The listing builds one solid part. Answer for the finished solid, in the listing's coordinates (mm). Coordinates: 2 decimals unless noted, no trailing zeros. Order: outer loops, then holes, each group sorted by start corner. A loop starts at its lowest first (then second) coordinate and runs counter-clockwise, first axis right, second up.
from build123d import *

# Parameters (mm, degrees)
F0_W     = 133.35
F0_H     = 73.025
F1_DEPTH = 3.175
F2_R     = 3.175
F3_DEPTH = 3.176
F4_R     = 3.96875
F5_DEPTH = 3.176


with BuildPart() as f1:
    # F0 (on Top) → F1 (new body)
    with BuildSketch(Plane.XY):
        with Locations((66.675, 36.5125)):
            Rectangle(F0_W, F0_H)
    extrude(amount=-F1_DEPTH)

    # F2 (on face) → F3 (cut, through all)
    with BuildSketch(Plane(origin=(0, 0, -3.175), x_dir=(1, 0, 0), z_dir=(0, 0, -1))):
        with Locations((28.575, -36.5125)):
            Circle(F2_R)
        with Locations((53.975, -36.5125)):
            Circle(F2_R)
        with Locations((79.375, -36.5125)):
            Circle(F2_R)
        with Locations((104.775, -36.5125)):
            Circle(F2_R)
    extrude(amount=-F3_DEPTH, mode=Mode.SUBTRACT)

    # F4 (on face) → F5 (cut, through all)
    with BuildSketch(Plane(origin=(0, 0, -3.175), x_dir=(1, 0, 0), z_dir=(0, 0, -1))):
        with Locations((28.575, -54.79161)):
            Circle(F4_R)
        with Locations((53.975, -54.79161)):
            Circle(F4_R)
        with Locations((79.375, -54.79161)):
            Circle(F4_R)
        with Locations((104.775, -54.79161)):
            Circle(F4_R)
        with Locations((104.775, -18.27911)):
            Circle(F4_R)
        with Locations((79.375, -18.27911)):
            Circle(F4_R)
        with Locations((53.975, -18.27911)):
            Circle(F4_R)
        with Locations((28.575, -18.27911)):
            Circle(F4_R)
    extrude(amount=-F5_DEPTH, mode=Mode.SUBTRACT)


solid = f1.part
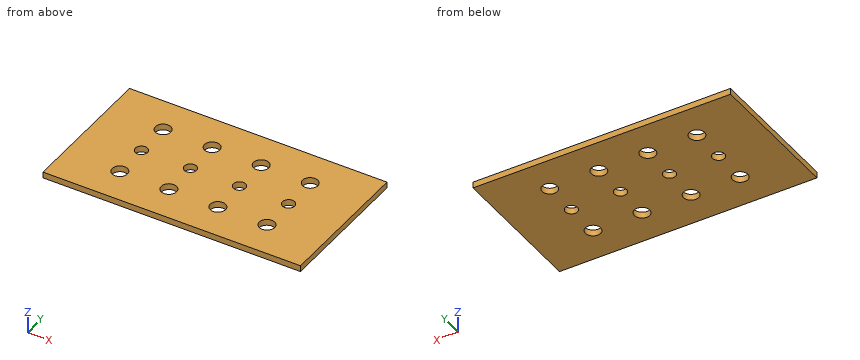
(1) Find section B-B on z = -1.45. Count the separate pieces of the cut face and the enclosed holes in it, then the cut area to 3 significant figures.
(2) Find section A-A on x = 28.5. Determine the outline of the cut face in (y, z) (3 decimals).
(3) Find the intervals of material crossed by probe 1 along Y at (x, z) = (104.5, -0.4) (3 decimals); probe 2 along Y at (x, z) = (27.5, -0.05) (1 decimal); probe 3 along X at (y, z) = (52.5, -2.9), in increasing order.
Resolved:
1. separate pieces: 1
1. enclosed holes: 12
1. area: 9,220 mm2
2. outline: (0, -3.175) - (14.311, -3.175) - (14.311, 0) - (0, 0) - close; (22.247, -3.175) - (33.338, -3.175) - (33.338, 0) - (22.247, 0) - close; (39.687, -3.175) - (50.824, -3.175) - (50.824, 0) - (39.687, 0) - close; (58.76, -3.175) - (73.025, -3.175) - (73.025, 0) - (58.76, 0) - close
3. probe 1: y = 0 to 14.32, 22.238 to 33.349, 39.676 to 50.832, 58.751 to 73.025
3. probe 2: y = 0 to 14.5, 22.1 to 33.5, 39.5 to 51, 58.6 to 73
3. probe 3: x = 0 to 25.33, 31.82 to 50.73, 57.22 to 76.13, 82.62 to 101.53, 108.02 to 133.35
